Check sheet for the modelled part. Datum: model origin and axes. Units: mm. A direction names the side the tool comes from. Round coordinates to 2 decimals unless told otherwise and drop trailing zeros. Order: outer loops, then holes, each group sorted by start corner. A loop starts at its lowest first (then second) coordinate and runs counter-clockwise, first axis right, second up.
Q1. Cross-section at D-D on y = 5.75. Record the cut outline in (x, z).
Q2. Cross-section at A-A on z = -14.25. Record the cut outline in (x, y).
Q3. Cross-section at C-C on x = 16. Record the cut outline in (y, z).
Q4. Scan lines: probe 1 along X at (y, z) = (10, -15); probe 2 along Z at (x, y) = (9, 18.25); probe 3 along X at (y, z) = (17.25, -1.5). Record each from-to range of solid material in increasing order.
Q5. Set-up check for faces 1 (the flat face through (10, 2, -15)), 2 (the flat face through (10, 15, -2)), 3 (the flat face through (17.9, -1, -2)), 4 (the flat face through (20, 15, -3)), 5 (the flat face through (10.1, -1, -25)): record each of +Z, -Z, +X, -X, +Y, -Y from which the full face is reachable in a straight line by a thin tool's end or side.
Q6. Depth check by flat-ended pin: P1, Ø10, axis at x = 22, z = -8, coming from the -Y side; P2, Ø1.7, axis at y = -1, z = -24.5, coming from the +X side; P3, Ø2, axis at x = 13.5, y = 5.5, coming from the +Z side. Enter the tip coordinate at first touch or a pass-through.
Q7. Mould release check, pull along Z, two halves, no side actions. Record for faces 6 (the flat face through (14, 11, -2)), 7 (the flat face through (14, 2, -11)), 8 (the flat face through (14, 1, 1)): +Z half, -Z half, draft (parallel to the pull), parting line (faces both ways), or undercut.
Q8. Cross-section at B-B on y = 14. Record the cut outline in (x, z).
from build123d import *

# Parameters (mm, degrees)
BOSS_EXTRUDE1_DEPTH = 28
SKETCH2_W           = 24
SKETCH2_H           = 24
CUT_EXTRUDE1_DEPTH  = 24
CUT_EXTRUDE2_REACH  = 47.706
SKETCH3_W           = 8
SKETCH3_H           = 8
CUT_EXTRUDE3_REACH  = 47.706
SKETCH4_W           = 8
SKETCH4_H           = 8
BOSS_EXTRUDE2_DEPTH = 3.9


with BuildPart() as part:
    # Sketch1 → Boss-Extrude1 (new body)
    with BuildSketch(Plane(origin=(0, 0, 0), x_dir=(0, 0, -1), z_dir=(1, 0, 0))):
        Polygon((0, 0), (0, 27), (3, 27), (27, 3), (27, 0), align=None)
    extrude(amount=BOSS_EXTRUDE1_DEPTH)

    # Sketch2 → Cut-Extrude1 (cut)
    with BuildSketch(Plane(origin=(0, 0, -27), x_dir=(-1, 0, 0), z_dir=(0, 0, -1))):
        with Locations((-14, 15)):
            Rectangle(SKETCH2_W, SKETCH2_H)
    extrude(amount=-CUT_EXTRUDE1_DEPTH, mode=Mode.SUBTRACT)

    # Sketch3 → Cut-Extrude2 (cut, up to next)
    with BuildSketch(Plane(origin=(0, 0, -3), x_dir=(-1, 0, 0), z_dir=(0, 0, -1)), mode=Mode.PRIVATE) as cut_extrude2_sk1:
        with Locations((-14, 15)):
            Rectangle(SKETCH3_W, SKETCH3_H)
    cut_extrude2_tool1 = extrude(cut_extrude2_sk1.sketch, amount=-CUT_EXTRUDE2_REACH, mode=Mode.PRIVATE) & part.part
    add(cut_extrude2_tool1.solids().sort_by_distance((14, 15, -3))[0], mode=Mode.SUBTRACT)

    # Sketch4 → Cut-Extrude3 (cut, up to next)
    with BuildSketch(Plane(origin=(0, 3, 0), x_dir=(1, 0, 0), z_dir=(0, 1, 0)), mode=Mode.PRIVATE) as cut_extrude3_sk1:
        with Locations((14, 15)):
            Rectangle(SKETCH4_W, SKETCH4_H)
    cut_extrude3_tool1 = extrude(cut_extrude3_sk1.sketch, amount=-CUT_EXTRUDE3_REACH, mode=Mode.PRIVATE) & part.part
    add(cut_extrude3_tool1.solids().sort_by_distance((14, 3, -15))[0], mode=Mode.SUBTRACT)

    # Sketch5 → Boss-Extrude2 (add, symmetric)
    with BuildSketch(Plane(origin=(14, 0, 0), x_dir=(0, 0, -1), z_dir=(1, 0, 0))):
        Polygon((27, 0), (24.878679656, -2.121320344), (23.464466094, -0.707106781), (24.171572875, 0), align=None)
        Polygon((2.121320344, -2.121320344), (0.707106781, -0.707106781), (1.414213562, 0), (4.242640687, 0), align=None)
        Polygon((0, 1.414213562), (-0.707106781, 0.707106781), (-2.121320344, 2.121320344), (0, 4.242640687), align=None)
        Polygon((-0.707106781, 23.464466094), (-2.121320344, 24.878679656), (0, 27), (0, 24.171572875), align=None)
    extrude(amount=BOSS_EXTRUDE2_DEPTH, both=True)


solid = part.part
Results found:
1. outline: (0, -24.25) - (2, -24.25) - (2, -3) - (26, -3) - (26, -24.25) - (28, -24.25) - (28, 0) - (0, 0) - close
2. outline: (0, 0) - (10, 0) - (10, 3) - (2, 3) - (2, 15.75) - (0, 15.75) - close; (18, 0) - (28, 0) - (28, 15.75) - (26, 15.75) - (26, 3) - (18, 3) - close
3. outline: (-2.12, -24.88) - (0, -27) - (3, -27) - (3, -19) - (0, -19) - (0, -24.17) - (-0.71, -23.46) - close; (-2.12, -2.12) - (0, -4.24) - (0, -11) - (3, -11) - (3, -3) - (11, -3) - (11, 0) - (4.24, 0) - (2.12, 2.12) - (0.71, 0.71) - (1.41, 0) - (0, 0) - (0, -1.41) - (-0.71, -0.71) - close; (19, -3) - (27, -3) - (27, 0) - (24.88, 2.12) - (23.46, 0.71) - (24.17, 0) - (19, 0) - close
4. probe 1: x = 0 to 2, 26 to 28
4. probe 2: z = -3 to 0
4. probe 3: x = 0 to 10, 18 to 28
5. face 1: +Y, -Y
5. face 2: +Z, -Z
5. face 3: +Z, -Z, +X, -Y
5. face 4: -Z, +Y
5. face 5: +Z, -Z, -X, -Y
6. P1: stops at y = 0
6. P2: stops at x = 17.9
6. P3: stops at z = 0
7. face 6: draft
7. face 7: undercut
7. face 8: +Z half
8. outline: (0, -16) - (2, -16) - (2, -3) - (10, -3) - (10, 0) - (0, 0) - close; (18, -3) - (26, -3) - (26, -16) - (28, -16) - (28, 0) - (18, 0) - close
